Autodesk Inventor part; units mm, degrees
ref_plane "YZ Plane" through (0, 0, 0) normal (1, 0, 0) x (0, 1, 0)
ref_plane "XZ Plane" through (0, 0, 0) normal (0, 1, 0) x (-1, 0, 0)
ref_plane "XY Plane" through (0, 0, 0) normal (0, 0, 1) x (1, 0, 0)
sketch "Skizze1" plane through (0, 0, 0) normal (0, 0, 1) x (1, 0, 0)
  circle A0 centre (0, 0) radius 3.5
  dimension "d0" = 7
extrude "Extrusion1" add sketch "Skizze1" along normal blind 5
sketch "Skizze2" plane through (0, 0, 0) normal (0, 0, -1) x (-1, 0, 0)
  circle A0 centre (0, 0) radius 2
  dimension "d3" = 4
extrude "Extrusion2" add sketch "Skizze2" along normal blind 1
sketch "Skizze3" plane through (0, 0, 5) normal (0, 0, 1) x (1, 0, 0)
  point P0 (0, 0)
hole "Bohrung1" at (0, 0, 5) direction (0, 0, -1) diameter 6 depth 3 tip angle 118
sketch "Skizze4" plane through (0, 0, -1) normal (0, 0, -1) x (-1, 0, 0)
  circle A0 centre (0, 0) radius 1
  dimension "d13" = 2
extrude "Extrusion3" add sketch "Skizze4" along normal blind 2
chamfer "Fase1" distance 1 angle 45 1 edges at (1, 0, -3)
properties part number "Wrist_EncoderMagnetMount" material "Messing, weicher Gelbton"
Verification items for the finished model (mm, model axes). A direction names the side the tool comes from. Round coordinates to 2 decimals unless told otherwise and drop trailing zeros. Order: outer loops, then holes, each group sorted by start corner. A loop starts at its lowest first (then second) coordinate and runs counter-clockwise, first axis right, second up. Notation, with made-up numbers: (-2, 9) - (18, 9) arc R11 ccw to (18, 22) - close; hole circle Ø11 at (-31, 22.5). An arc over 180 degrees is marked (long way). Use CSV: the item, a comma, the result in double quotes. Start each with the question number.
1) Go/stop test with flat-tipped pins: P1, Ø3, axis at x = -0.5, y = -2, coming from the -Z side; P2, Ø3, axis at x = -2, z = -0.5, coming from the +Y side. Record where each tip stops, or that it passes through.
2) Mould release check, pull along X, two halves, no side actions. Record for faces 3 (the cylindrical face through (3.233, 1.341, 2.465)), 4 (the conical face through (-0.46, -0.24, 0.51)), 5 (the flat face through (2, -2, 0)), 6 (the cylindrical face through (0, 3, 3)): +X half, -X half, draft (parallel to the pull), parting line (faces both ways), or undercut.
3) Section check A-A, the plane z = 3. Record the cut outline in (x, y).
4) Section check B-B, the plane z = -1.25. Record the cut outline in (x, y), plus the area to 3 significant figures.
5) Access from +Z, -Z, +X, -X, +Y, -Y to the whole of each face (thin tool, end or side, straight path). Record for faces 1 (the flat face through (3, 1, 5)), 2 (the cylindrical face through (0.217, 0.976, -1.493)).
6) Thickness scan on L1, parallel to Y at x = 0, z = 3.3; L2, parallel to Y at x = 1, z = 3.75; L3, parallel to X at y = -2, z = 2.75. Record the ranges inside material, lowest first.
7) Section check C-C, the plane z = 1. Record the cut outline in (x, y), plus the area to 3 significant figures.
Answers:
1,P1,"stops at z = -2.44"
1,P2,"stops at y = 3.45"
2,face 3,"parting line"
2,face 4,"undercut"
2,face 5,"draft"
2,face 6,"undercut"
3,outline,"circle Ø7 at (0, 0); hole circle Ø6 at (0, 0)"
4,outline,"circle Ø2 at (0, 0)"
4,area,"3.14 mm²"
5,face 1,"+Z, +X, -X, +Y, -Y"
5,face 2,"-Z"
6,L1,"y = -3.5 to -3, 3 to 3.5"
6,L2,"y = -3.35 to -2.83, 2.83 to 3.35"
6,L3,"x = -2.87 to -2.24, 2.24 to 2.87"
7,outline,"circle Ø7 at (0, 0); hole circle Ø2.67 at (0, 0)"
7,area,"32.9 mm²"
